from build123d import *

# Parameters (mm, degrees)
BOSS_EXTRUDE1_DEPTH      = 10
BOSS_EXTRUDE1_DEPTH_BACK = 10
SKETCH1_W                = 78
SKETCH1_H                = 67
FILLET1_R                = 2.5
SKETCH2_W                = 2.5
SKETCH2_H                = 10
BOSS_EXTRUDE2_DEPTH      = 5
FILLET2_R                = 0.5


with BuildPart() as part:
    # Sketch1 → Boss-Extrude1 (new, two sides: drawn at the far end of the back side and taken through both)
    with BuildSketch(Plane(origin=(0, 0, 0), x_dir=(1, 0, 0), z_dir=(0, 1, 0)).offset(-BOSS_EXTRUDE1_DEPTH_BACK)):
        Rectangle(SKETCH1_W, SKETCH1_H)
    extrude(amount=BOSS_EXTRUDE1_DEPTH + BOSS_EXTRUDE1_DEPTH_BACK)

    # Fillet1
    fillet1_edges = [part.edges().sort_by_distance(p)[0] for p in [
        (-39, -10, 0),
        (39, 10, 0),
        (0, 10, -33.5),
        (0, -10, 33.5),
        (-39, 10, 0),
        (0, 10, 33.5),
        (39, -10, 0),
        (0, -10, -33.5),
        (39, 0, 33.5),
        (-39, 0, 33.5),
        (-39, 0, -33.5),
        (39, 0, -33.5),
    ]]
    fillet(fillet1_edges, radius=FILLET1_R)

    # Sketch2 → Boss-Extrude2 (add)
    with BuildSketch(Plane(origin=(0, 0, -33.5), x_dir=(-1, 0, 0), z_dir=(0, 0, -1))):
        with Locations((35.25, 0)):
            Rectangle(SKETCH2_W, SKETCH2_H)
    extrude(amount=BOSS_EXTRUDE2_DEPTH)

    # Fillet2
    fillet2_edges = [part.edges().sort_by_distance(p)[0] for p in [
        (-34, -5, -36),
        (-35.25, -5, -38.5),
        (-34, 0, -38.5),
        (-35.25, 5, -38.5),
        (-34, 5, -36),
        (-36.5, -5, -36),
        (-36.5, 0, -38.5),
        (-36.5, 5, -36),
    ]]
    fillet(fillet2_edges, radius=FILLET2_R)
    fillet2_2_edges = [part.edges().sort_by_distance(p)[0] for p in [
        (-34, 0, -33.5),
        (-35.25, -5, -33.5),
        (-35.25, 5, -33.5),
        (-36.5, 0, -33.5),
        (-36.353553391, 4.853553391, -33.5),
        (-36.353553391, -4.853553391, -33.5),
        (-34.146446609, 4.853553391, -33.5),
        (-34.146446609, -4.853553391, -33.5),
    ]]
    fillet(fillet2_2_edges, radius=FILLET2_R)


solid = part.part
Work out the finished part from the listing and answer in its coordinate system (mm). A direction names the side the tool comes from. Give positions to 0.01 mm unless a question says otherwise; leave off trailing zeros. Loops run counter-clockwise (first coordinate to the right, second up) from the corner with the lowest first, then second, coordinate; pieces in that order, holes last. Notation, with made-up numbers: (12, 50.5) -> (56, 50.5) arc R18 cw to (56, 71.5) -> close; hole circle Ø4 at (-24.5, 46). An arc over 180 degrees is marked (long way). Use a Markdown table: item, result. Add a question column.
1) The part is cut by section B-B, the plane x = -25.5. Determine the outline of the cut face in (y, z), plus the area to 3 significant figures.
2) Each of these flat-tipped pins is pushed along its axis until it touches: P1, Ø1, axis at x = 14.5, y = -1, coming from the -Z side; P2, Ø2, axis at y = 0.5, z = -36, coming from the +X side; P3, Ø1.2, axis at y = 0, z = -35, coming from the -X side. Where does it stop, or does it pass through?
3) For a pull along X with two mould halves and no side action, classify faces 4 (the cylindrical face through (38, 0, 33)), 5 (the cylindrical face through (1, 9, 33)), 6 (the cylindrical face through (-38.287, 9.248, -0.434)) as +X half, -X half, draft (parallel to the pull), parting line (faces both ways), or undercut.
4) Which of the six approach directions +Z, -Z, +X, -X, +Y, -Y give full straight-line access (tool end or side, diameter ignored) to faces 1 (the flat face through (-36.5, 0, -36)), 2 (the cylindrical face through (1, -9, 33)), 3 (the flat face through (-34, 0, -36))?
5) Consider line 1 along Z through (x, y) = (-31.5, -1); line 2 along X through (y, z) = (8.75, -18.5); line 3 along X through (y, z) = (-8, 3). Determine where each line is inside the solid, lowest interval first.
6) The part is cut by section A-A, the plane y = 3.25. Determine the outline of the cut face in (x, z).
Reported:
| question | item | result |
|---|---|---|
| 1 | outline | (-10, -31) arc R2.5 ccw to (-7.5, -33.5) -> (7.5, -33.5) arc R2.5 ccw to (10, -31) -> (10, 31) arc R2.5 ccw to (7.5, 33.5) -> (-7.5, 33.5) arc R2.5 ccw to (-10, 31) -> close |
| 1 | area | 1,330 mm^2 |
| 2 | P1 | stops at z = -33.5 |
| 2 | P2 | stops at x = -34 |
| 2 | P3 | stops at x = -36.5 |
| 3 | face 4 | +X half |
| 3 | face 5 | draft |
| 3 | face 6 | -X half |
| 4 | face 1 | -Z, -X, +Y, -Y |
| 4 | face 2 | +Z, +X, -X, -Y |
| 4 | face 3 | -Z, +X, +Y, -Y |
| 5 | line 1 | z = -33.5 to 33.5 |
| 5 | line 2 | x = -38.67 to 38.67 |
| 5 | line 3 | x = -38.95 to 38.95 |
| 6 | outline | (-39, -31) arc R2.5 ccw to (-36.92, -33.47) arc R0.5 cw to (-36.5, -33.96) -> (-36.5, -38) arc R0.5 ccw to (-36, -38.5) -> (-34.5, -38.5) arc R0.5 ccw to (-34, -38) -> (-34, -34) arc R0.5 cw to (-33.5, -33.5) -> (36.5, -33.5) arc R2.5 ccw to (39, -31) -> (39, 31) arc R2.5 ccw to (36.5, 33.5) -> (-36.5, 33.5) arc R2.5 ccw to (-39, 31) -> close |
